```python
from build123d import *

# Parameters (mm, degrees)
BOSS_EXTRUDE1_DEPTH = 1000
SKETCH2_R           = 2.125
CUT_EXTRUDE1_DEPTH  = 5
LPATTERN1_COUNT     = 10
LPATTERN1_PITCH     = 100


with BuildPart() as part:
    # Sketch1 → Boss-Extrude1 (new body)
    with BuildSketch(Plane(origin=(0, 0, 0), x_dir=(1, 0, 0), z_dir=(0, 1, 0))):
        with BuildLine():
            Line((15, -22.5), (-15, -22.5))
            Line((-15, -22.5), (-15, -18.5))
            Line((-15, -18.5), (-6, -18.5))
            Line((-6, -18.5), (-6, -11.5))
            Line((-6, -11.5), (-3.25, -5.04356025))
            ThreePointArc((-3.25, -5.04356025), (0, 6), (3.25, -5.04356025))
            Line((3.25, -5.04356025), (6, -11.5))
            Line((6, -11.5), (6, -18.5))
            Line((6, -18.5), (15, -18.5))
            Line((15, -18.5), (15, -22.5))
        make_face()
    extrude(amount=BOSS_EXTRUDE1_DEPTH)

    # Sketch2 → Cut-Extrude1 (cut, through all)
    with BuildSketch(Plane(origin=(0, 0, 18.5), x_dir=(-1, 0, 0), z_dir=(0, 0, -1))):
        with Locations((-11, 950)):
            Circle(SKETCH2_R)
        with Locations((11, 950)):
            Circle(SKETCH2_R)
    cut_extrude1 = extrude(amount=-CUT_EXTRUDE1_DEPTH, mode=Mode.SUBTRACT)

    # LPattern1: Cut-Extrude1 ×10
    with Locations(*[(0, -i * LPATTERN1_PITCH, 0) for i in range(1, LPATTERN1_COUNT)]):
        add(cut_extrude1, mode=Mode.SUBTRACT)


solid = part.part
```
For this review, take the finished solid that the model builds, in its own axes (mm). Coordinates: 2 decimals unless noted, no trailing zeros. Write each loop counter-clockwise with the first axis right and the second up, starting at its lowest first coordinate (ties: lowest second). Pieces come first, ordered by that corner, then holes.
(1) For pin 1 Ø7 at (x, y) = (11, 250) entering from -Z; pin 2 Ø2 at (y, z) = (524, 14) entering from -X; pin 3 Ø12 at (y, z) = (179, 3.5) entering from +X, all flat-tipped, find the tip position at first contact; note any pin that passes through.
(2) Wall thickness on probe 1 along X at (y, z) = (350, 19.7) (3 decimals); probe 2 along X at (y, z) = (665, -1.5); probe 3 along X at (y, z) = (267, 17): over which ranges is each line inside the solid? List them lowest first.
(3) Add section A-A on y = 274. Give the boundary of the cut face in (x, z).
Answer sheet:
1. pin 1: stops at z = 18.5
1. pin 2: stops at x = -6
1. pin 3: stops at x = 6
2. probe 1: x = -15 to -13.125, -8.875 to 8.875, 13.125 to 15
2. probe 2: x = -5.81 to 5.81
2. probe 3: x = -6 to 6
3. outline: (-15, 18.5) - (-6, 18.5) - (-6, 11.5) - (-3.25, 5.04) arc R6 ccw (long way) to (3.25, 5.04) - (6, 11.5) - (6, 18.5) - (15, 18.5) - (15, 22.5) - (-15, 22.5) - close
